```python
from build123d import *

# Parameters (mm, degrees)
SKETCH1_W           = 12.7
SKETCH1_H           = 8.89
BOSS_EXTRUDE1_DEPTH = 76.2
SKETCH2_W           = 8.89
SKETCH2_H           = 6.35
BOSS_EXTRUDE2_DEPTH = 6.35
SKETCH3_W           = 8.89
SKETCH3_H           = 6.35
BOSS_EXTRUDE3_DEPTH = 6.35
SKETCH4_W           = 6.35
SKETCH4_H           = 8.89
BOSS_EXTRUDE4_DEPTH = 15.24
SKETCH7_W           = 6.35
SKETCH7_H           = 8.89
BOSS_EXTRUDE5_DEPTH = 15.24
SKETCH8_R           = 3.302
CUT_EXTRUDE2_DEPTH  = 35.306
SKETCH6_R           = 3.302
CUT_EXTRUDE3_DEPTH  = 33.528


with BuildPart() as part:
    # Sketch1 → Boss-Extrude1 (new body)
    with BuildSketch(Plane(origin=(0, 0, 0), x_dir=(1, 0, 0), z_dir=(0, 1, 0))):
        with Locations((6.35, 4.445)):
            Rectangle(SKETCH1_W, SKETCH1_H)
    extrude(amount=BOSS_EXTRUDE1_DEPTH)

    # Sketch2 → Boss-Extrude2 (add)
    with BuildSketch(Plane(origin=(12.7, 0, 0), x_dir=(0, 0, -1), z_dir=(1, 0, 0))):
        with Locations((4.445, 3.175)):
            Rectangle(SKETCH2_W, SKETCH2_H)
        with Locations((4.445, 73.025)):
            Rectangle(SKETCH2_W, SKETCH2_H)
    extrude(amount=BOSS_EXTRUDE2_DEPTH)

    # Sketch3 → Boss-Extrude3 (add)
    with BuildSketch(Plane.ZY):
        with Locations((-4.445, 3.175)):
            Rectangle(SKETCH3_W, SKETCH3_H)
        with Locations((-4.445, 73.025)):
            Rectangle(SKETCH3_W, SKETCH3_H)
    extrude(amount=BOSS_EXTRUDE3_DEPTH)

    # Sketch4 → Boss-Extrude4 (add)
    with BuildSketch(Plane(origin=(0, 76.2, 0), x_dir=(1, 0, 0), z_dir=(0, 1, 0))):
        with Locations((-3.175, 4.445)):
            Rectangle(SKETCH4_W, SKETCH4_H)
        with Locations((15.875, 4.445)):
            Rectangle(SKETCH4_W, SKETCH4_H)
    extrude(amount=BOSS_EXTRUDE4_DEPTH)

    # Sketch7 → Boss-Extrude5 (add)
    with BuildSketch(Plane.XZ):
        with Locations((-3.175, -4.445)):
            Rectangle(SKETCH7_W, SKETCH7_H)
        with Locations((15.875, -4.445)):
            Rectangle(SKETCH7_W, SKETCH7_H)
    extrude(amount=BOSS_EXTRUDE5_DEPTH)

    # Sketch8 → Cut-Extrude2 (cut)
    with BuildSketch(Plane(origin=(19.05, 0, 0), x_dir=(0, 0, -1), z_dir=(1, 0, 0))):
        with Locations((4.445, -10.16)):
            Circle(SKETCH8_R)
    extrude(amount=-CUT_EXTRUDE2_DEPTH, mode=Mode.SUBTRACT)

    # Sketch6 → Cut-Extrude3 (cut)
    with BuildSketch(Plane(origin=(19.05, 0, 0), x_dir=(0, 0, -1), z_dir=(1, 0, 0))):
        with Locations((4.445, 86.36)):
            Circle(SKETCH6_R)
    extrude(amount=-CUT_EXTRUDE3_DEPTH, mode=Mode.SUBTRACT)


solid = part.part
```
Geometry check sheet. Reference: the model listing, model coordinates, mm. A direction names the side the tool comes from. Coordinates: 2 decimals unless noted, no trailing zeros. Write each loop counter-clockwise with the first axis right and the second up, starting at its lowest first coordinate (ties: lowest second). Pieces come first, ordered by that corner, then holes. Notation, with made-up numbers: M 29.25,3 L 55.25,3 A24 ccw 55.25,34 Z; hole C 52.5,37.5 d5. An arc over 180 degrees is marked long. Use one line per item in the form item = value. Start each with the question number.
1) Set-up check for faces 1 (the flat face through (16, -15.24, -4)), 2 (the flat face through (12.7, 82, -4)), 3 (the flat face through (6, 0, -5)), 4 (the flat face through (16, 69.85, -4)), 5 (the flat face through (-3, 6.35, -5)): record each of +Z, -Z, +X, -X, +Y, -Y from which the full face is reachable in a straight line by a thin tool's end or side.
2) Section check C-C on x = 6.75. Enter the section's corners in (y, z).
3) Section check A-A on x = -1.75. Enter the section's corners in (y, z) (3 decimals), and give its area (3 significant figures).
4) Section check D-D on y = 44. Enter the section's corners in (x, z), and give its area (3 significant figures).
5) Thickness scan on probe 1 along Y at (x, z) = (18.25, -0.5); probe 2 along X at (y, z) = (-8, -7); probe 3 along Y at (x, z) = (13.75, -1.75). Record the ranges inside material, lowest first. Write a range as from..to.
6) Go/stop test with flat-tipped pins: pin 1 Ø2 at (y, z) = (32.5, -2.5) entering from -X; pin 2 Ø3 at (x, z) = (3, -6.5) entering from -Y; pin 3 Ø4.5 at (x, z) = (8.5, -6.5) entering from +Y. Record where each tip stops, or that it passes through.
7) Section check B-B on y = -10.16. Enter the section's corners in (x, z).
8) Release check for a two-part mould opening along Z. For faces 6 (the flat face through (-6.35, -4, -5)), 7 (the flat face through (6, 39, 0)), 8 (the cylindrical face through (-3.131, -7.376, -6.22)) record: pulls with the +Z half, pulls with the -Z half, needs draft (parallel to the pull), parting line crosses it, or undercut.
Responses:
q1.face_1 = +Z, -Z, +X, -X, -Y
q1.face_2 = +Z, -Z, +Y
q1.face_3 = +Z, -Z, -Y
q1.face_4 = +Z, -Z, +X
q1.face_5 = +Z, -Z, -X
q2.outline = M 0,-8.89 L 76.2,-8.89 L 76.2,0 L 0,0 Z
q3.outline = M -15.24,-8.89 L 6.35,-8.89 L 6.35,0 L -15.24,0 Z; M 69.85,-8.89 L 91.44,-8.89 L 91.44,0 L 69.85,0 Z; hole C -10.16,-4.445 d6.604; hole C 86.36,-4.445 d6.604
q3.area = 315 mm2
q4.outline = M 0,-8.89 L 12.7,-8.89 L 12.7,0 L 0,0 Z
q4.area = 113 mm2
q5.probe_1 = -15.24..6.35, 69.85..91.44
q5.probe_2 = -6.35..0, 12.7..19.05
q5.probe_3 = -15.24..-12.07, -8.25..6.35, 69.85..84.45, 88.27..91.44
q6.pin_1 = 0
q6.pin_2 = 0
q6.pin_3 = 76.2
q7.outline = M -6.35,-8.89 L 0,-8.89 L 0,-7.75 L -6.35,-7.75 Z; M -6.35,-1.14 L 0,-1.14 L 0,0 L -6.35,0 Z; M 12.7,-8.89 L 19.05,-8.89 L 19.05,-7.75 L 12.7,-7.75 Z; M 12.7,-1.14 L 19.05,-1.14 L 19.05,0 L 12.7,0 Z
q8.face_6 = needs draft
q8.face_7 = pulls with the +Z half
q8.face_8 = undercut
